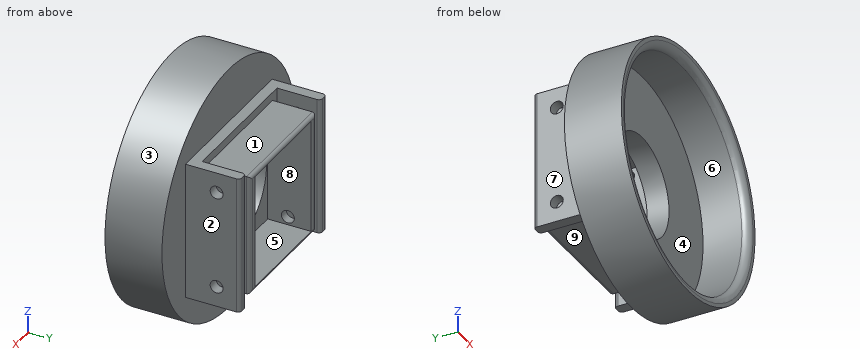
from build123d import *

# Parameters (mm, degrees)
F0_R     = 34.038
F0_R_2   = 31.038
F0_W     = 38.1
F0_H     = 38.1
F0_R_3   = 13.7
F1_DEPTH = 3
F2_DEPTH = 3
F3_DEPTH = 15.7
F4_R     = 2
F5_W     = 3
F5_H     = 38.1
F5_W_2   = 33.528
F5_H_2   = 33.528
F5_W_3   = 28.528
F5_H_3   = 31.528
F6_DEPTH = 15
F7_R     = 0.99999
F8_R     = 1.778
F9_DEPTH = 56.089


# Not quite as in the source:
# - a fillet or chamfer is up to 0.001 mm smaller than in the source, because OpenCascade refuses the exact size
# - a feature names something its author has since deleted; it is built from what else it names


with BuildPart() as f1:
    # F0 (on Front) → F1 (new body)
    with BuildSketch(Plane.XZ):
        Circle(F0_R)
        Circle(F0_R_2, mode=Mode.SUBTRACT)
        Circle(F0_R_2)
        Rectangle(F0_W, F0_H, mode=Mode.SUBTRACT)
        Rectangle(F0_W, F0_H)
        Circle(F0_R_3, mode=Mode.SUBTRACT)
    extrude(amount=F1_DEPTH)

    # F0 (on Front) → F2 (join)
    with BuildSketch(Plane.XZ):
        Rectangle(F0_W, F0_H)
        Circle(F0_R_3, mode=Mode.SUBTRACT)
    extrude(amount=-F2_DEPTH)

    # F0 (on Front) → F3 (join)
    with BuildSketch(Plane.XZ):
        Circle(F0_R)
        Circle(F0_R_2, mode=Mode.SUBTRACT)
    extrude(amount=F3_DEPTH)

    # F4
    f4_edges = [f1.edges().sort_by_distance(p)[0] for p in [
        (-31.038, -15.7, 0),
    ]]
    fillet(f4_edges, radius=F4_R)

    # F5 (on Front) → F6 (join)
    with BuildSketch(Plane.XZ):
        with Locations((-20.55, 0)):
            Rectangle(F5_W, F5_H)
        with Locations((20.55, 0)):
            Rectangle(F5_W, F5_H)
        Rectangle(F5_W_2, F5_H_2)
        Rectangle(F5_W_3, F5_H_3, mode=Mode.SUBTRACT)
    extrude(amount=-F6_DEPTH)

    # F7 (radius 1 in the source; OpenCascade refuses exactly that, so slightly less here)
    f7_edges = [f1.edges().sort_by_distance(p)[0] for p in [
        (-19.05, 15, 0),
        (-16.764, 15, 0),
        (19.05, 15, 0),
        (16.764, 15, 0),
        (0, 15, 16.764),
        (0, 15, -16.764),
        (22.05, 15, 0),
        (-22.05, 15, 0),
    ]]
    fillet(f7_edges, radius=F7_R)

    # F8 (on face) → F9 (cut, through all)
    with BuildSketch(Plane(origin=(-22.05, 0, 0), x_dir=(0, -1, 0), z_dir=(-1, 0, 0))):
        with Locations((-8.5796158184, 13.4703841816)):
            Circle(F8_R)
        with Locations((-8.5796158184, -13.4703841816)):
            Circle(F8_R)
    extrude(amount=-F9_DEPTH, mode=Mode.SUBTRACT)


solid = f1.part
Design review of the part built by this model. Coordinates are the model's own, in mm. Face numbers are marked on the shaded views. A direction names the side the tool comes from. Coordinates: 2 decimals unless noted, no trailing zeros. Order: outer loops, then holes, each group sorted by start corner. A loop starts at its lowest first (then second) coordinate and runs counter-clockwise, first axis right, second up.
Item 1: Take a section at A-A, the plane y = 5. Write out the cut boundary in (x, z).
Item 2: For pin 1 Ø16.5 at (x, y) = (7, 4) entering from +Z; pin 2 Ø9 at (y, z) = (9.5, 4) entering from +X; pin 3 Ø4 at (x, z) = (-11, 8.5) entering from -Y; pin 4 Ø23 at (x, z) = (-5.5, 1) entering from +Y, all flat-tipped, find the tip position at first contact; note any pin that passes through.
Item 3: Take a section at C-C, the plane y = 1. Write out the cut boundary in (x, z), then the cut area to 3 significant figures.
Item 4: The part is to be moulded in two halves that separate along Z. For the marked faces 6, 7, 8 and 9, say which applies: pulls with the +Z half, pulls with the -Z half, needs draft (parallel to the pull), parting line crosses it, or undercut.
Item 5: For the marked faces 1, 2, 3, 4 and 5, list the 3-axis set-ups (+Z, -Z, +X, -X, +Y, -Y) from which the entire face can be reached by the end or side of a thin tool; tool diameter is ignored.
Item 6: For line 1 (X direction, y = 13.5, z = 5.5); line 2 (Z direction, x = -9.5, y = 4); line 3 (X direction, y = 12, z = -19), list the stretches that pass through material, from the lowest coordinate up.
Item 7: Take a section at D-D, the plane y = -9. Write out the cut boundary in (x, z), then the cut area to 3 significant figures.
The answers:
1. outline: (-22.05, -19.05) - (-19.05, -19.05) - (-19.05, 19.05) - (-22.05, 19.05) - close; (-16.76, -16.76) - (16.76, -16.76) - (16.76, 16.76) - (-16.76, 16.76) - close; (19.05, -19.05) - (22.05, -19.05) - (22.05, 19.05) - (19.05, 19.05) - close; hole (-14.26, -15.76) - (14.26, -15.76) - (14.26, 15.76) - (-14.26, 15.76) - close
2. pin 1: stops at z = 34.04
2. pin 2: stops at x = 22.05
2. pin 3: stops at y = -3
2. pin 4: stops at y = 15
3. outline: (-22.05, -19.05) - (22.05, -19.05) - (22.05, 19.05) - (-22.05, 19.05) - close; hole circle Ø27.4 at (0, 0)
3. area: 1,090 mm2
4. face 6: undercut
4. face 7: needs draft
4. face 8: undercut
4. face 9: pulls with the -Z half
5. face 1: +Z, +Y
5. face 2: +Z, -Z, +X, +Y
5. face 3: +Y, -Y
5. face 4: -Y
5. face 5: +Y
6. line 1: x = -22.05 to -19.05, -16.76 to -14.26, 14.26 to 16.76, 19.05 to 22.05
6. line 2: z = -16.76 to -15.76, 15.76 to 16.76
6. line 3: x = -22.05 to -19.05, 19.05 to 22.05
7. outline: circle Ø68.08 at (0, 0); hole circle Ø62.08 at (0, 0)
7. area: 613 mm2
